from build123d import *

# Parameters (mm, degrees)
SKETCH1_R           = 10
BOSS_EXTRUDE1_DEPTH = 100
SKETCH2_R           = 7.5
BOSS_EXTRUDE2_DEPTH = 40
SKETCH3_W           = 15
SKETCH3_H           = 4
CUT_EXTRUDE1_DEPTH  = 14
SKETCH4_R           = 2
CUT_EXTRUDE2_DEPTH  = 70
SKETCH5_R           = 4
CUT_EXTRUDE3_DEPTH  = 36
SKETCH6_R           = 4
CUT_EXTRUDE4_DEPTH  = 36


with BuildPart() as part:
    # Sketch1 → Boss-Extrude1 (new body, symmetric)
    with BuildSketch(Plane.XY):
        Circle(SKETCH1_R)
    extrude(amount=BOSS_EXTRUDE1_DEPTH, both=True)

    # Sketch2 → Boss-Extrude2 (add)
    with BuildSketch(Plane(origin=(0, 0, 0), x_dir=(1, 0, 0), z_dir=(0, 1, 0))):
        with Locations((0, 60)):
            Circle(SKETCH2_R)
        with Locations((0, -60)):
            Circle(SKETCH2_R)
    extrude(amount=BOSS_EXTRUDE2_DEPTH)

    # Sketch3 → Cut-Extrude1 (cut)
    with BuildSketch(Plane(origin=(0, 40, 0), x_dir=(1, 0, 0), z_dir=(0, 1, 0))):
        with Locations((0, -60)):
            Rectangle(SKETCH3_W, SKETCH3_H)
        with Locations((0, 60)):
            Rectangle(SKETCH3_W, SKETCH3_H)
    extrude(amount=-CUT_EXTRUDE1_DEPTH, mode=Mode.SUBTRACT)

    # Sketch4 → Cut-Extrude2 (cut, symmetric)
    with BuildSketch(Plane.XY):
        with Locations((0, 34)):
            Circle(SKETCH4_R)
    extrude(amount=CUT_EXTRUDE2_DEPTH, both=True, mode=Mode.SUBTRACT)

    # Sketch5 → Cut-Extrude3 (cut)
    with BuildSketch(Plane(origin=(0, 0, -100), x_dir=(-1, 0, 0), z_dir=(0, 0, -1))):
        with Locations((0, 34)):
            Circle(SKETCH5_R)
    extrude(amount=-CUT_EXTRUDE3_DEPTH, mode=Mode.SUBTRACT)

    # Sketch6 → Cut-Extrude4 (cut)
    with BuildSketch(Plane.XY.offset(100)):
        with Locations((0, 34)):
            Circle(SKETCH6_R)
    extrude(amount=-CUT_EXTRUDE4_DEPTH, mode=Mode.SUBTRACT)


solid = part.part
Could you check a few things on this model? Use its own coordinates, in mm. A direction names the side the tool comes from. Round coordinates to 2 decimals unless told otherwise and drop trailing zeros. Write each loop counter-clockwise with the first axis right and the second up, starting at its lowest first coordinate (ties: lowest second). Pieces come first, ordered by that corner, then holes. Notation, with made-up numbers: (72.25, 66.25) - (77.25, 66.25) arc R21 ccw to (77.25, 84.25) - close; hole circle Ø8 at (55.25, -24). An arc over 180 degrees is marked (long way). Put each result on its own line as item: value. Start each with the question number.
(1) I want a section at C-C, the plane y = 4. Please give me the cut outline in (x, z).
(2) Thinking about a two-plate mould opening in X: for faces 6 (the cylindrical face through (-2.17, -9.76, 1.4)), 7 (the flat face through (-0.1, 31.5, -62)), 8 (the cylindrical face through (0, 32, -63)), which applies, released by +X, released by -X, zero draft, split by the parting line, or undercut?
(3) I want a section at A-A, the plane x = 0. Give the number of separate pieces and of enclosed holes in the cut face, plus the area to 3 significant figures.
(4) For faces 1 (the flat face through (0, 40, -64)), 2 (the cylindrical face through (0, 32, 63)), 3 (the flat face through (-0.1, 31.5, 62)), 4 (the cylindrical face through (6.93, 23.07, -57.13)), 5 (the cylindrical face through (4, 34, -65)), which set-ups out of +Z, -Z, +X, -X, +Y, -Y let a thin tool reach every point of the face, with its end or its side?
(5) I need wall thicknesses on probe 1 along Y at (x, z) = (0, -65.4); probe 2 along Z at (x, y) = (0, 24.5); probe 3 along Z at (x, y) = (-6.5, 30). Which ranges of each line are inside material? Lowest first, please.
(6) I want a section at B-B, the plane z = 60. Please give me the cut outline in (x, y), plus the area to 3 significant figures.
(7) Will these pins go through, and if not, where does the flat tip stop? pin 1 (4 mm diameter, centred on x = 7, z = 41, fed in from -Y); pin 2 (5 mm diameter, centred on x = -4.5, z = 79, fed in from -Y); pin 3 (10 mm diameter, centred on x = 7.5, y = 27.5, fed in from -Z).
(8) I want a section at D-D, the plane z = 26. Please give me the cut outline in (x, y).
Here are the results:
1. outline: (-9.17, -100) - (9.17, -100) - (9.17, 100) - (-9.17, 100) - close
2. face 6: split by the parting line
2. face 7: zero draft
2. face 8: undercut
3. separate pieces: 5
3. enclosed holes: 0
3. area: 4,670 mm^2
4. face 1: +Z, -Z, +X, -X, +Y
4. face 2: +Z, -Z
4. face 3: +X, -X, +Y
4. face 4: +Y
4. face 5: -Z
5. probe 1: y = -10 to 30, 38 to 40
5. probe 2: z = -67.5 to -52.5, 52.5 to 67.5
5. probe 3: z = -63.74 to -62, -58 to -56.26, 56.26 to 58, 62 to 63.74
6. outline: (-7.5, 6.61) arc R10 ccw (long way) to (7.5, 6.61) - (7.5, 26) - (-7.5, 26) - close
6. area: 570 mm^2
7. pin 1: stops at y = -8.66
7. pin 2: stops at y = -9.8
7. pin 3: stops at z = -67.07
8. outline: circle Ø20 at (0, 0)
